from build123d import *

# Parameters (mm, degrees)
SKETCH1_W           = 40
SKETCH1_H           = 38
SKETCH1_R           = 2.474873734
SKETCH1_R_2         = 1.5
SKETCH1_R_3         = 2
BOSS_EXTRUDE3_DEPTH = 2
SKETCH1_5_W         = 40
SKETCH1_5_H         = 2
BOSS_EXTRUDE4_DEPTH = 47
FILLET1_R           = 20
FILLET2_R           = 1
SKETCH2_R           = 1.5
CUT_EXTRUDE2_DEPTH  = 47


with BuildPart() as part:
    # Sketch1 → Boss-Extrude3 (new body)
    with BuildSketch(Plane(origin=(0, 0, 0), x_dir=(1, 0, 0), z_dir=(0, 1, 0))):
        with Locations((0, -1)):
            Rectangle(SKETCH1_W, SKETCH1_H)
        with Locations(Location((-15.5, -12, 0), (0, 0, 270))):
            Circle(SKETCH1_R, mode=Mode.SUBTRACT)
        with Locations(Location((15.5, -12, 0), (0, 0, 270))):
            Circle(SKETCH1_R_2, mode=Mode.SUBTRACT)
        with Locations(Location((16.5, -4, 0), (0, 0, 270))):
            Circle(SKETCH1_R_3, mode=Mode.SUBTRACT)
        with Locations(Location((-15.5, 12, 0), (0, 0, 270))):
            Circle(SKETCH1_R_3, mode=Mode.SUBTRACT)
        with Locations(Location((16.5, 4, 0), (0, 0, 270))):
            Circle(SKETCH1_R_3, mode=Mode.SUBTRACT)
        with Locations(Location((15.5, 12, 0), (0, 0, 270))):
            Circle(SKETCH1_R_2, mode=Mode.SUBTRACT)
    extrude(amount=BOSS_EXTRUDE3_DEPTH)

    # Sketch1<5> → Boss-Extrude4 (add)
    with BuildSketch(Plane(origin=(0, 0, 0), x_dir=(1, 0, 0), z_dir=(0, 1, 0))):
        with Locations((0, 19)):
            Rectangle(SKETCH1_5_W, SKETCH1_5_H)
    extrude(amount=BOSS_EXTRUDE4_DEPTH)

    # Fillet1
    fillet1_edges = [part.edges().sort_by_distance(p)[0] for p in [
        (20, 47, -19),
        (-20, 47, -19),
    ]]
    fillet(fillet1_edges, radius=FILLET1_R - 0.0001)  # a hair under: the kernel refuses the full size

    # Fillet2
    fillet2_edges = [part.edges().sort_by_distance(p)[0] for p in [
        (0, 0, -20),
    ]]
    fillet(fillet2_edges, radius=FILLET2_R)

    # Sketch2 → Cut-Extrude2 (cut)
    with BuildSketch(Plane.XY.offset(-18)):
        with Locations((-14, 25)):
            Circle(SKETCH2_R)
        with Locations((-7, 37.124355653)):
            Circle(SKETCH2_R)
        with Locations((7, 37.124355653)):
            Circle(SKETCH2_R)
        with Locations((14, 25)):
            Circle(SKETCH2_R)
        with Locations((7, 12.875644347)):
            Circle(SKETCH2_R)
        with Locations((-7, 12.875644347)):
            Circle(SKETCH2_R)
        with BuildLine():
            Line((6, 31.5), (6, 18.5))
            ThreePointArc((6, 18.5), (0, 12.5), (-6, 18.5))
            Line((-6, 18.5), (-6, 31.5))
            ThreePointArc((-6, 31.5), (0, 37.5), (6, 31.5))
        make_face()
    extrude(amount=-CUT_EXTRUDE2_DEPTH, mode=Mode.SUBTRACT)


solid = part.part
Model file for the job. Use its own axes, mm. A direction names the side the tool comes from. Round coordinates to 2 decimals unless told otherwise and drop trailing zeros. Order: outer loops, then holes, each group sorted by start corner. A loop starts at its lowest first (then second) coordinate and runs counter-clockwise, first axis right, second up.
(1) Pull direction Y, two halves, no side cores. Call faces 4 (the face through (0, 2, 1)), 5 (the face through (15.57, 0.99, -13.5)), 6 (the face through (5.81, 11.96, -18.99)): released by +Y, released by -Y, zero draft, split by the parting line, or undercut.
(2) Band-saw the part on A-A (y = 21). List the corners of the cut face in (x, z).
(3) 3-axis set-ups, long thin cutter, end or side, ignore diameter. For faces 1 (the face through (14.297, 40.986, -19.014)), 2 (the face through (-9, 24, -18)), 3 (the face through (0.1, 12.5, -19)): which of +Z, -Z, +X, -X, +Y, -Y reach the whole face in a straight line?
(4) Band-saw the part on C-C (z = -4). List the corners of the cut face in (x, y), then the cut area to 3 significant figures.
(5) Band-saw the part on B-B (z = -12). List the corners of the cut face in (x, y), then the cut area to 3 significant figures.
(6) Pin check, flat tips, straight feed: pin 1 (20 mm diameter, centred on x = -10, y = 25, fed in from +Z); pin 2 (5 mm diameter, centred on x = -16, z = -5.5, fed in from +Y). Stop position of each tip, or through.
(7) Drill centre lines: line 1 (X direction, y = 1, z = 12); line 2 (X direction, y = 1, z = 4); line 3 (Y direction, x = -12, z = 11). Where is each one in solid material? Low to high.
(8) Band-saw the part on D-D (x = 7). List the corners of the cut face in (y, z), then the cut area to 3 significant figures.
Verdict:
1. face 4: released by +Y
1. face 5: zero draft
1. face 6: undercut
2. outline: (-20, -20) - (-6, -20) - (-6, -18) - (-20, -18) - close; (6, -20) - (20, -20) - (20, -18) - (6, -18) - close
3. face 1: +Z, -Z, +X, +Y
3. face 2: +Z, +X, -X, +Y
3. face 3: +Z, -Z
4. outline: (-20, 0) - (14.5, 0) - (14.5, 2) - (-20, 2) - close; (18.5, 0) - (20, 0) - (20, 2) - (18.5, 2) - close
4. area: 72.0 mm2
5. outline: (-20, 0) - (-17.5, 0) - (-17.5, 2) - (-20, 2) - close; (-13.5, 0) - (14, 0) - (14, 2) - (-13.5, 2) - close; (17, 0) - (20, 0) - (20, 2) - (17, 2) - close
5. area: 66.0 mm2
6. pin 1: stops at z = -18
6. pin 2: stops at y = 2
7. line 1: x = -20 to -17.97, -13.03 to 14, 17 to 20
7. line 2: x = -20 to 14.5, 18.5 to 20
7. line 3: y = 0 to 2
8. outline: (0, -19) arc R1 ccw to (1, -20) - (11.38, -20) - (11.38, -18) - (2, -18) - (2, 20) - (0, 20) - close; (14.38, -20) - (35.62, -20) - (35.62, -18) - (14.38, -18) - close; (38.62, -20) - (45.74, -20) - (45.74, -18) - (38.62, -18) - close
8. area: 155 mm2
